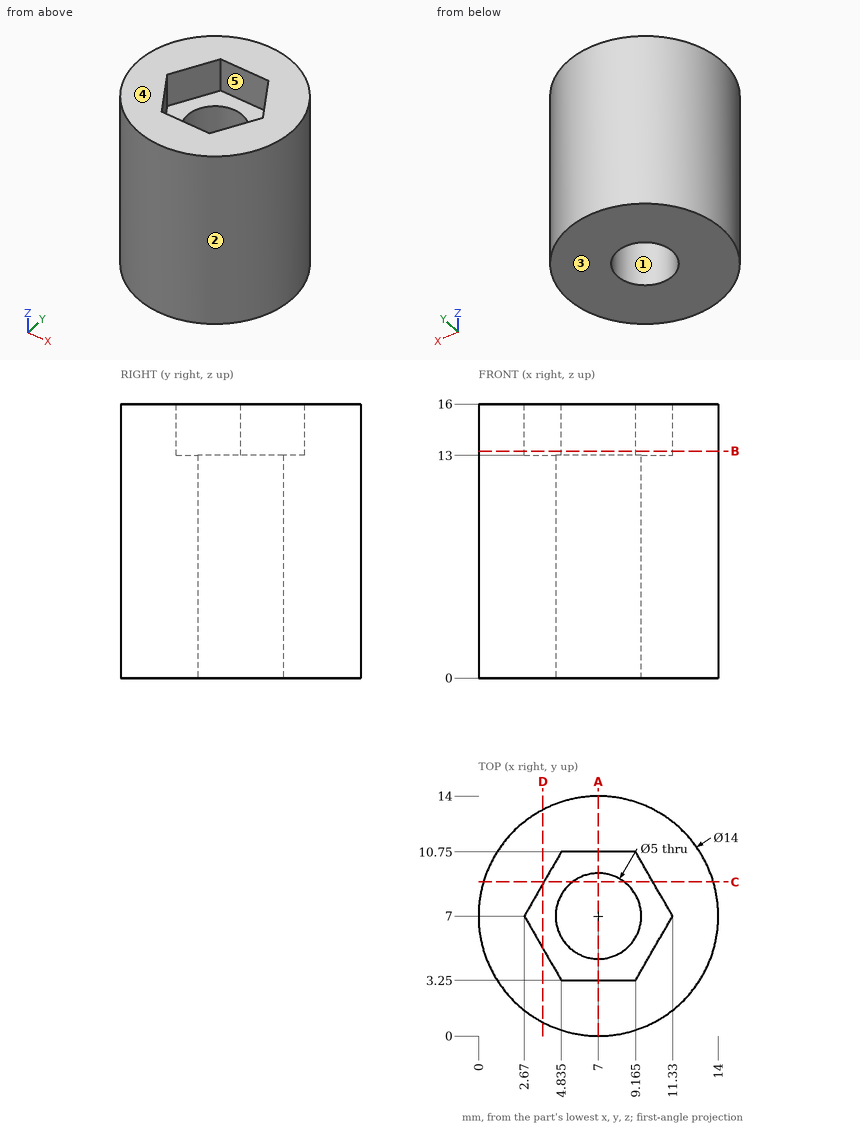
The figure shows three views and two pictorial views of one solid part (mm, origin at its lowest corner). Answer the questions. A direction names the side the tool comes from. Coordinates: 2 decimals unless noted, no trailing zeros. Write each loop counter-clockwise with the first axis right and the second up, starting at its lowest first coordinate (ties: lowest second). Pieces come first, ordered by that corner, then holes. Notation, with made-up numbers: (42, -30) -> (100, -30) arc R28 ccw to (100, -10) -> close; hole circle Ø9 at (16, 83.5). An arc over 180 degrees is marked (long way). Return JSON: item names as keys, results as strings.
1. A cutting plane is placed at A-A (x = 7). Determine the outline of the cut face in (y, z).
Found:
{"outline": "(0, 0) -> (4.5, 0) -> (4.5, 13) -> (3.25, 13) -> (3.25, 16) -> (0, 16) -> close; (9.5, 0) -> (14, 0) -> (14, 16) -> (10.75, 16) -> (10.75, 13) -> (9.5, 13) -> close"}
2. A cutting plane is placed at D-D (x = 3.75). Determine the outline of the cut face in (y, z).
Found:
{"outline": "(0.8, 0) -> (13.2, 0) -> (13.2, 16) -> (8.87, 16) -> (8.87, 13) -> (5.13, 13) -> (5.13, 16) -> (0.8, 16) -> close"}
3. A tool of negligible diameter and unlimited length cuts with its end or side. For the marked faces 4 and 5, from which of +Z, -Z, +X, -X, +Y, -Y can it reach the whole face along a straight path? Write none if from no direction.
Found:
{"face 4": "+Z, +X, -X, +Y, -Y", "face 5": "+Z"}
4. Find the intervals of material crossed by line 1 along Y through (x, z) = (7, 5.5); line 2 along Y through (x, z) = (3, 14.25) (1 decimal); line 3 along Z through (x, y) = (9.75, 9.25), in increasing order. Write a range as from..to.
Found:
{"line 1": "0..4.5, 9.5..14", "line 2": "1.3..6.4, 7.6..12.7", "line 3": "0..13"}
5. Each of these flat-tipped pins is pushed along its axis until it touches: P1, Ø6, axis at x = 2, y = 12.5, coming from the +Z side; P2, Ø8, axis at y = 2, z = 6, coming from the +X side; P3, Ø6, axis at x = 7, y = 6.5, coming from the +Z side; P4, Ø4, axis at y = 1.5, z = 7.5, coming from the +X side. Where does it stop, or does it pass through?
Found:
{"P1": "z = 16", "P2": "x = 13.93", "P3": "z = 13", "P4": "x = 13.06"}
6. Determine the mould class of the marked faces 1, 2 and 3 for opening direction Y: pulls with the +Y half, pulls with the -Y half, needs draft (parallel to the pull), parting line crosses it, or undercut.
Found:
{"face 1": "undercut", "face 2": "parting line crosses it", "face 3": "needs draft"}
7. A cutting plane is placed at C-C (y = 9). Determine the outline of the cut face in (x, z), and give its area (3 significant figures).
Found:
{"outline": "(0.29, 0) -> (5.5, 0) -> (5.5, 13) -> (3.82, 13) -> (3.82, 16) -> (0.29, 16) -> close; (8.5, 0) -> (13.71, 0) -> (13.71, 16) -> (10.18, 16) -> (10.18, 13) -> (8.5, 13) -> close", "area": "157 mm2"}
8. A cutting plane is placed at B-B (z = 13.25). Determine the outline of the cut face in (x, y) (3 decimals).
Found:
{"outline": "circle Ø14 at (7, 7); hole (2.67, 7) -> (4.835, 3.25) -> (9.165, 3.25) -> (11.33, 7) -> (9.165, 10.75) -> (4.835, 10.75) -> close"}
